Check sheet for the modelled part. Datum: model origin and axes. Units: mm. A direction names the side the tool comes from. Give positions to 0.01 mm unless a question says otherwise; leave off trailing zeros. Order: outer loops, then holes, each group sorted by start corner. A loop starts at its lowest first (then second) coordinate and runs counter-clockwise, first axis right, second up.
```python
from build123d import *

# Parameters (mm, degrees)
SKETCH1_R           = 2.75
BOSS_EXTRUDE1_DEPTH = 5
SKETCH2_R           = 2.75
BOSS_EXTRUDE2_DEPTH = 5
BOSS_EXTRUDE3_START = -20
BOSS_EXTRUDE3_DEPTH = 20
FILLET1_R           = 5


with BuildPart() as part:
    # Sketch1 → Boss-Extrude1 (new body)
    with BuildSketch(Plane.XY):
        with BuildLine():
            ThreePointArc((7.840741737, 145.091301473), (5.644042596, 150.394602332), (0.340741737, 152.591301473))
            Line((0.340741737, 152.591301473), (-9.659258263, 152.591301473))
            Line((-9.659258263, 152.591301473), (-9.659258263, 167.591301473))
            Line((-9.659258263, 167.591301473), (-20.400000003, 167.591301473))
            Line((-20.400000003, 167.591301473), (-20.4, 122.320508076))
            ThreePointArc((-20.4, 122.320508076), (-20.045628593, 119.628790007), (-19.006664199, 117.120508076))
            Line((-19.006664199, 117.120508076), (3.628732497, 77.914850942))
            Line((3.628732497, 77.914850942), (12.930487699, 83.285221812))
            Line((12.930487699, 83.285221812), (5.430487699, 96.275602869))
            Line((5.430487699, 96.275602869), (14.090741737, 101.275602869))
            ThreePointArc((14.090741737, 101.275602869), (17.585185434, 105.829650559), (16.835932265, 111.520793398))
            Line((16.835932265, 111.520793398), (7.840741737, 127.100920417))
            Line((7.840741737, 127.100920417), (7.840741737, 145.091301473))
        make_face()
        with Locations((10.340741737, 107.770793398)):
            Circle(SKETCH1_R, mode=Mode.SUBTRACT)
        with Locations((0.340741737, 125.091301473)):
            Circle(SKETCH1_R, mode=Mode.SUBTRACT)
        with Locations((0.340741737, 145.091301473)):
            Circle(SKETCH1_R, mode=Mode.SUBTRACT)
    extrude(amount=BOSS_EXTRUDE1_DEPTH)



with BuildPart() as body_2:
    # Sketch2 → Boss-Extrude2 (new body)
    with BuildSketch(Plane(origin=(0, 0, -10), x_dir=(-1, 0, 0), z_dir=(0, 0, -1))):
        with BuildLine():
            Line((-14.090741737, 101.275602869), (-5.430487699, 96.275602869))
            Line((-5.430487699, 96.275602869), (-12.930487699, 83.285221812))
            Line((-12.930487699, 83.285221812), (-3.628732497, 77.914850942))
            Line((-3.628732497, 77.914850942), (19.006664199, 117.120508076))
            ThreePointArc((19.006664199, 117.120508076), (20.045628593, 119.628790007), (20.4, 122.320508076))
            Line((20.4, 122.320508076), (20.400000003, 167.591301473))
            Line((20.400000003, 167.591301473), (9.659258263, 167.591301473))
            Line((9.659258263, 167.591301473), (9.659258263, 152.591301473))
            Line((9.659258263, 152.591301473), (-0.340741737, 152.591301473))
            ThreePointArc((-0.340741737, 152.591301473), (-5.644042596, 150.394602332), (-7.840741737, 145.091301473))
            Line((-7.840741737, 145.091301473), (-7.840741737, 127.100920417))
            Line((-7.840741737, 127.100920417), (-16.835932265, 111.520793398))
            ThreePointArc((-16.835932265, 111.520793398), (-17.585185434, 105.829650559), (-14.090741737, 101.275602869))
        make_face()
        with Locations(Location((-10.340741737, 107.770793398, 0), (0, 0, 180))):
            Circle(SKETCH2_R, mode=Mode.SUBTRACT)
        with Locations(Location((-0.340741737, 125.091301473, 0), (0, 0, 180))):
            Circle(SKETCH2_R, mode=Mode.SUBTRACT)
        with Locations(Location((-0.340741737, 145.091301473, 0), (0, 0, 180))):
            Circle(SKETCH2_R, mode=Mode.SUBTRACT)
    extrude(amount=BOSS_EXTRUDE2_DEPTH)


with BuildPart() as part_1:
    add(part.part)

    add(body_2.part)  # Boss-Extrude3 merges body 2
    # Sketch3 → Boss-Extrude3 (add)
    with BuildSketch(Plane.XY.offset(5).offset(BOSS_EXTRUDE3_START)):
        with BuildLine():
            Line((-0.701394522, 75.414850943), (3.628732497, 77.914850942))
            Line((3.628732497, 77.914850942), (-19.006664199, 117.120508076))
            ThreePointArc((-19.006664199, 117.120508076), (-20.045628593, 119.628790007), (-20.4, 122.320508076))
            Line((-20.4, 122.320508076), (-20.400000003, 167.591301473))
            Line((-20.400000003, 167.591301473), (-25.400000003, 167.591301473))
            Line((-25.400000003, 167.591301473), (-25.4, 122.320508076))
            ThreePointArc((-25.4, 122.320508076), (-24.875257725, 118.334694781), (-23.336791218, 114.620508076))
            Line((-23.336791218, 114.620508076), (-0.701394522, 75.414850943))
        make_face()
    extrude(amount=BOSS_EXTRUDE3_DEPTH)

    # Fillet1
    fillet1_edges = [part_1.edges().sort_by_distance(p)[0] for p in [
        (5.430487699, 96.275602869, 2.5),
        (12.930487699, 83.285221812, 2.5),
        (-9.659258263, 167.591301473, 2.5),
        (-9.659258263, 152.591301473, 2.5),
        (-0.701394522, 75.414850943, -5),
        (-25.400000003, 167.591301473, -5),
        (5.430487699, 96.275602869, -12.5),
        (12.930487699, 83.285221812, -12.5),
        (-9.659258263, 167.591301473, -12.5),
        (-9.659258263, 152.591301473, -12.5),
    ]]
    fillet(fillet1_edges, radius=FILLET1_R - 0.0001)  # a hair under: the kernel refuses the full size


solid = part_1.part
```
(1) Cross-section at D-D on y = 140. Enter the section's corners in (x, z), then the cut area to 3 significant figures.
Response values:
outline: (-25.4, -15) - (7.84, -15) - (7.84, -10) - (-20.4, -10) - (-20.4, 0) - (7.84, 0) - (7.84, 5) - (-25.4, 5) - close
area: 382 mm2
(2) Release check for a two-part mould opening along X. For faces 5 (the face through (-13.41, 97.43, -5.14)), 6 (the face through (-0.017, 147.818, 2.465)), 7 (the face through (10.944, 83.874, 2.535)), 8 (the face through (-0.255, 122.407, 2.465)) record: released by +X, released by -X, zero draft, split by the parting line, or undercut.
Response values:
face 5: released by -X
face 6: undercut
face 7: released by +X
face 8: undercut
(3) Material ranges on L1, parallel to Z at x = -17, y = 158.5; L2, parallel to X at y = 123, z = 1.5; L3, parallel to X at y = 133, z = -7.75, recorded low to high.
Response values:
L1: z = -15 to -10, 0 to 5
L2: x = -25.4 to -1.45, 2.13 to 10.21
L3: x = -25.4 to -20.4
(4) Set-up check for faces 1 (the face through (-20.4, 145, -5)), 2 (the face through (9.163, 89.811, -12.465)), 3 (the face through (7.841, 136, 2)), 4 (the face through (-0.017, 122.365, -12.465)): record each of +Z, -Z, +X, -X, +Y, -Y from which the full face is reachable in a straight line by a thin tool's end or side.
Response values:
face 1: +X, +Y
face 2: +Z, -Z, +X
face 3: +Z, -Z, +X, +Y
face 4: +Z, -Z
(5) Cross-section at A-A on y = 123.5. Enter the section's corners in (x, z), then the cut area to 3 significant figures.
Response values:
outline: (-25.4, -15) - (-1.9, -15) - (-1.9, -10) - (-20.4, -10) - (-20.4, 0) - (-1.9, 0) - (-1.9, 5) - (-25.4, 5) - close; (2.58, -15) - (9.92, -15) - (9.92, -10) - (2.58, -10) - close; (2.58, 0) - (9.92, 0) - (9.92, 5) - (2.58, 5) - close
area: 358 mm2
(6) Gauge pin test, flat ends, axial feed: pin 1 Ø1.5 at (y, z) = (160, -11.5) entering from +X; pin 2 Ø3 at (y, z) = (101, 0.5) entering from +X; pin 3 Ø2.5 at (y, z) = (138.5, 3) entering from +X. Record the tip position at first contact, or that the pin passes through.
Response values:
pin 1: stops at x = -9.66
pin 2: stops at x = 15.68
pin 3: stops at x = 7.84
(7) Cross-section at C-C on z = 1.75. Enter the section's corners in (x, y), then the cut area to 3 significant figures.
Response values:
outline: (-25.4, 122.32) arc R15.4 ccw to (-23.34, 114.62) - (-3.2, 79.74) arc R5 ccw to (3.63, 77.91) - (8.6, 80.79) arc R5 ccw to (10.43, 87.62) - (7.93, 91.95) arc R5 cw to (9.76, 98.78) - (14.09, 101.28) arc R7.5 ccw to (16.84, 111.52) - (7.84, 127.1) - (7.84, 145.09) arc R7.5 ccw to (0.34, 152.59) - (-4.66, 152.59) arc R5 cw to (-9.66, 157.59) - (-9.66, 162.59) arc R5 ccw to (-14.66, 167.59) - (-20.4, 167.59) arc R5 ccw to (-25.4, 162.59) - close; hole circle Ø5.5 at (0.34, 125.09); hole circle Ø5.5 at (0.34, 145.09); hole circle Ø5.5 at (10.34, 107.77)
area: 2,360 mm2
